Work out the finished part from the listing and answer in its coordinate system (mm). A direction names the side the tool comes from. Give positions to 0.01 mm unless a question says otherwise; leave off trailing zeros. Loops run counter-clockwise (first coordinate to the right, second up) from the corner with the lowest first, then second, coordinate; pieces in that order, holes last. Notation, with made-up numbers: (-5, 22) - (10, 22) arc R18 cw to (10, 55) - close; hole circle Ø7 at (62, 43.5). An arc over 180 degrees is marked (long way). Use one line per item in the form item = value. Start each with the question number.
from build123d import *

# Parameters (mm, degrees)
EXTRUDE10_DEPTH          = 31.75
EXTRUDE10_DEPTH_BACK     = 31.75
SKETCH10_R               = 7.14375
BOSS_EXTRUDE7_DEPTH      = 31.75
BOSS_EXTRUDE7_DEPTH_BACK = 31.75
SKETCH31_R               = 7.14375
BOSS_EXTRUDE8_DEPTH      = 10.715625
CHAMFER2_SIZE            = 0.508


with BuildPart() as part:
    # Sketch10 → Extrude10 (new, two sides: drawn at the far end of the back side and taken through both)
    with BuildSketch(Plane.XY.offset(-EXTRUDE10_DEPTH_BACK)):
        Circle(SKETCH10_R)
    extrude(amount=EXTRUDE10_DEPTH + EXTRUDE10_DEPTH_BACK)



with BuildPart() as body_2:
    # Sketch31 → Boss-Extrude7 (new, two sides: drawn at the far end of the back side and taken through both)
    with BuildSketch(Plane(origin=(0, 0, 0), x_dir=(1, 0, 0), z_dir=(0, 1, 0)).offset(-BOSS_EXTRUDE7_DEPTH_BACK)):
        with Locations(Location((0, 0, 0), (0, 0, 270))):
            Circle(SKETCH31_R)
    extrude(amount=BOSS_EXTRUDE7_DEPTH + BOSS_EXTRUDE7_DEPTH_BACK)


with BuildPart() as part_1:
    add(part.part)

    add(body_2.part)  # Boss-Extrude8 merges body 2
    # Sketch32 → Boss-Extrude8 (add, symmetric)
    with BuildSketch(Plane(origin=(0, 0, 0), x_dir=(0, 0, -1), z_dir=(1, 0, 0))):
        Polygon((9.286875, -22.420499577), (22.420499577, -9.286875), (22.420499577, 9.286875), (9.286875, 22.420499577), (-9.286875, 22.420499577), (-22.420499577, 9.286875), (-22.420499577, -9.286875), (-9.286875, -22.420499577), align=None)
    extrude(amount=BOSS_EXTRUDE8_DEPTH, both=True)

    # Chamfer2
    chamfer2_edges = [part_1.edges().sort_by_distance(p)[0] for p in [
        (0, -31.75, -7.14375),
        (0, 31.75, -7.14375),
        (-7.14375, 0, -31.75),
        (-7.14375, 0, 31.75),
    ]]
    chamfer(chamfer2_edges, length=CHAMFER2_SIZE)


solid = part_1.part
1) Flat-ended cylindrical pins translate along their axes: pin 1 Ø3 at (x, z) = (8, -7.5) entering from -Y; pin 2 Ø6 at (x, y) = (-1, -11) entering from -Z; pin 3 Ø12 at (x, y) = (-3, -21) entering from -Z. Find the tip coordinate at first contact, or state that the pin passes through.
2) Find the intervals of material crossed by probe 1 along Z at (x, y) = (-9, -4); probe 2 along Z at (x, y) = (8, -18), in increasing order.
3) A cutting plane is placed at A-A (y = 0). Give the vertices of the cut face in (x, z), plus the area to 3 significant figures.
4) A tool of negligible diameter and unlimited length cuts with its end or side. For faces 1 (the flat face through (7.3, -0.1, -22.42)), 2 (the flat face through (7.3, -22.42, 0.1)), 3 (the flat face through (7.3, 22.42, -0.1)), from which of +Z, -Z, +X, -X, +Y, -Y can it reach the whole face along a straight path? Write none if from no direction.
5) A cutting plane is placed at D-D (x = 8). Give the vertices of the cut face in (y, z).
Answer sheet:
q1.pin_1 = -22.42
q1.pin_2 = -22.42
q1.pin_3 = -16.71
q2.probe_1 = -22.42 to 22.42
q2.probe_2 = -13.71 to 13.71
q3.outline = (-10.72, -22.42) - (-7.14, -22.42) - (-7.14, -31.24) - (-6.64, -31.75) - (6.64, -31.75) - (7.14, -31.24) - (7.14, -22.42) - (10.72, -22.42) - (10.72, 22.42) - (7.14, 22.42) - (7.14, 31.24) - (6.64, 31.75) - (-6.64, 31.75) - (-7.14, 31.24) - (-7.14, 22.42) - (-10.72, 22.42) - close
q3.area = 1,230 mm²
q4.face_1 = -Z
q4.face_2 = -Y
q4.face_3 = +Y
q5.outline = (-22.42, -9.29) - (-9.29, -22.42) - (9.29, -22.42) - (22.42, -9.29) - (22.42, 9.29) - (9.29, 22.42) - (-9.29, 22.42) - (-22.42, 9.29) - close
